Work out the finished part from the listing and answer in its coordinate system (mm). Round coordinates to 2 decimals unless told otherwise and drop trailing zeros. Loops run counter-clockwise (first coordinate to the right, second up) from the corner with the lowest first, then second, coordinate; pieces in that order, holes last. Notation, with made-up numbers: (75, -1.75) - (81, -1.75) arc R23 cw to (81, 37.25) - close; hole circle Ø8 at (-28, 52). An arc over 180 degrees is marked (long way). Return JSON: item names as keys, results as strings.
from build123d import *

# Parameters (mm, degrees)
F0_W     = 109
F0_H     = 70
F0_R     = 1.1
F0_R_2   = 6.3
F1_DEPTH = 1
F2_W     = 53
F2_H     = 10.5
F3_DEPTH = 1
F5_DEPTH = 1
F6_R     = 1
F7_R     = 1.1
F7_W     = 40
F7_H     = 16.5
F7_R_2   = 10
F8_DEPTH = 1
F9_R     = 3


# Not quite as in the source:
# - a feature names something its author has since deleted; it is built from what else it names


with BuildPart() as f1:
    # F0 (on Top) → F1 (new body)
    with BuildSketch(Plane.XY):
        Rectangle(F0_W, F0_H)
        with Locations((-51.5, -26)):
            Circle(F0_R, mode=Mode.SUBTRACT)
        with Locations((-35.5, -26)):
            Circle(F0_R, mode=Mode.SUBTRACT)
        with Locations((-23.5, -21.5)):
            Circle(F0_R, mode=Mode.SUBTRACT)
        with BuildLine():
            ThreePointArc((-37.5, -14.5), (-37.7928932188, -15.2071067812), (-38.5, -15.5))
            Line((-38.5, -15.5), (-48.5, -15.5))
            ThreePointArc((-48.5, -15.5), (-49.2071067812, -15.2071067812), (-49.5, -14.5))
            Line((-49.5, -14.5), (-49.5, -8.5))
            ThreePointArc((-49.5, -8.5), (-49.2071067812, -7.7928932188), (-48.5, -7.5))
            Line((-48.5, -7.5), (-38.5, -7.5))
            ThreePointArc((-38.5, -7.5), (-37.7928932188, -7.7928932188), (-37.5, -8.5))
            Line((-37.5, -8.5), (-37.5, -14.5))
        make_face(mode=Mode.SUBTRACT)
        with Locations((23.5, -21.5)):
            Circle(F0_R, mode=Mode.SUBTRACT)
        with Locations((35.5, -26)):
            Circle(F0_R, mode=Mode.SUBTRACT)
        with Locations((51.5, -26)):
            Circle(F0_R, mode=Mode.SUBTRACT)
        with BuildLine():
            Line((38.5, -7.5), (48.5, -7.5))
            ThreePointArc((48.5, -7.5), (49.2071067812, -7.7928932188), (49.5, -8.5))
            Line((49.5, -8.5), (49.5, -14.5))
            ThreePointArc((49.5, -14.5), (49.2071067812, -15.2071067812), (48.5, -15.5))
            Line((48.5, -15.5), (38.5, -15.5))
            ThreePointArc((38.5, -15.5), (37.7928932188, -15.2071067812), (37.5, -14.5))
            Line((37.5, -14.5), (37.5, -8.5))
            ThreePointArc((37.5, -8.5), (37.7928932188, -7.7928932188), (38.5, -7.5))
        make_face(mode=Mode.SUBTRACT)
        with Locations((-43.5, 3.5)):
            Circle(F0_R_2, mode=Mode.SUBTRACT)
        with Locations((-51.5, 10)):
            Circle(F0_R, mode=Mode.SUBTRACT)
        with Locations((-35.5, 10)):
            Circle(F0_R, mode=Mode.SUBTRACT)
        with Locations((-23.5, 21.5)):
            Circle(F0_R, mode=Mode.SUBTRACT)
        with Locations((43.5, 3.5)):
            Circle(F0_R_2, mode=Mode.SUBTRACT)
        with Locations((35.5, 10)):
            Circle(F0_R, mode=Mode.SUBTRACT)
        with Locations((51.5, 10)):
            Circle(F0_R, mode=Mode.SUBTRACT)
        with Locations((23.5, 21.5)):
            Circle(F0_R, mode=Mode.SUBTRACT)
    extrude(amount=F1_DEPTH)

    # F2 (on face) → F3 (cut, through all)
    with BuildSketch(Plane.XY.offset(1)):
        with BuildLine():
            Line((-26.5, 35), (-54.5, 35))
            Line((-54.5, 35), (-54.5, 13))
            Line((-54.5, 13), (-28.5, 13))
            ThreePointArc((-28.5, 13), (-27.0857864376, 13.5857864376), (-26.5, 15))
            Line((-26.5, 15), (-26.5, 24.5))
            Line((-26.5, 24.5), (-26.5, 35))
        make_face()
        with Locations((0, 29.75)):
            Rectangle(F2_W, F2_H)
        with BuildLine():
            Line((54.5, 35), (26.5, 35))
            Line((26.5, 35), (26.5, 24.5))
            Line((26.5, 24.5), (26.5, 15))
            ThreePointArc((26.5, 15), (27.0857864376, 13.5857864376), (28.5, 13))
            Line((28.5, 13), (54.5, 13))
            Line((54.5, 13), (54.5, 35))
        make_face()
    extrude(amount=-F3_DEPTH, mode=Mode.SUBTRACT)

    # F4 (on face) → F5 (cut, through all)
    with BuildSketch(Plane.XY.offset(1)):
        Polygon((-54.5, -29), (-54.5, -35), (0, -35), (54.5, -35), (54.5, -29), (0, -29), align=None)
    extrude(amount=-F5_DEPTH, mode=Mode.SUBTRACT)

    # F6
    f6_edges = [f1.edges().sort_by_distance(p)[0] for p in [
        (-54.5, -29, 0.5),
        (54.5, -29, 0.5),
        (54.5, 13, 0.5),
        (26.5, 24.5, 0.5),
        (-26.5, 24.5, 0.5),
        (-54.5, 13, 0.5),
    ]]
    fillet(f6_edges, radius=F6_R)

    # F7 (on face) → F8 (cut, through all)
    with BuildSketch(Plane.XY.offset(1)):
        with Locations((-22.5, -10)):
            Circle(F7_R)
        with Locations((22.5, -10)):
            Circle(F7_R)
        with Locations((-22.5, 12.5)):
            Circle(F7_R)
        with Locations((22.5, 12.5)):
            Circle(F7_R)
        with Locations((0, -20.75)):
            Rectangle(F7_W, F7_H)
        with Locations((0, 6)):
            Circle(F7_R_2)
    extrude(amount=-F8_DEPTH, mode=Mode.SUBTRACT)

    # F9
    f9_edges = [f1.edges().sort_by_distance(p)[0] for p in [
        (-20, -29, 0.5),
        (-20, -12.5, 0.5),
        (20, -12.5, 0.5),
        (20, -29, 0.5),
    ]]
    fillet(f9_edges, radius=F9_R)


solid = f1.part
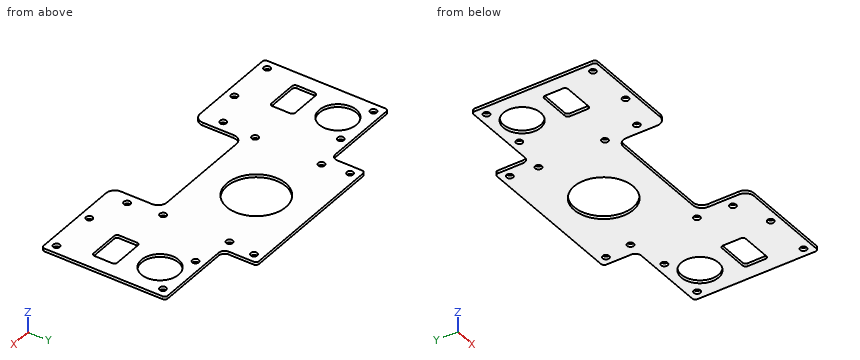
1) Section B-B (x = -51.5) is taken. Give the vertices of the cut face in (y, z).
Verdict:
{"outline": "(-29, 0) - (-27.1, 0) - (-27.1, 1) - (-29, 1) - close; (-24.9, 0) - (8.9, 0) - (8.9, 1) - (-24.9, 1) - close; (11.1, 0) - (13, 0) - (13, 1) - (11.1, 1) - close"}
2) Find the intervals of material crossed by L1, parallel to Y at x = 35.5, z = 0.75; L2, parallel to X at y = 22.5, z = 0.75; L3, parallel to X at y = -19, z = 0.9, in increasing order.
Verdict:
{"L1": "y = -29 to -27.1, -24.9 to 8.9, 11.1 to 13", "L2": "x = -26.5 to -23.96, -23.04 to 23.04, 23.96 to 26.5", "L3": "x = -54.5 to -20, 20 to 54.5"}
3) Section C-C (y = -17) is taken. Give the vertices of the cut face in (x, z), and give its area (3 significant figures).
Verdict:
{"outline": "(-54.5, 0) - (-20, 0) - (-20, 1) - (-54.5, 1) - close; (20, 0) - (54.5, 0) - (54.5, 1) - (20, 1) - close", "area": "69.0 mm2"}
4) Section D-D (y = 6) is taken. Give the vertices of the cut face in (x, z).
Verdict:
{"outline": "(-54.5, 0) - (-49.28, 0) - (-49.28, 1) - (-54.5, 1) - close; (-37.72, 0) - (-10, 0) - (-10, 1) - (-37.72, 1) - close; (10, 0) - (37.72, 0) - (37.72, 1) - (10, 1) - close; (49.28, 0) - (54.5, 0) - (54.5, 1) - (49.28, 1) - close"}
5) Flat-ended cylindrical pins translate along their axes: pin 1 (23 mm diameter, centred on x = 0, y = 6, fed in from +Z); pin 2 (0.5 mm diameter, centred on x = -45.5, z = 0.5, fed in from +Y). Find the tip coordinate at first contact, or state that the pin passes through.
Verdict:
{"pin 1": "stops at z = 1", "pin 2": "stops at y = 13"}
6) Section A-A (y = -10) is taken. Give the vertices of the cut face in (x, z), and give its area (3 significant figures).
Verdict:
{"outline": "(-54.5, 0) - (-49.5, 0) - (-49.5, 1) - (-54.5, 1) - close; (-37.5, 0) - (-23.6, 0) - (-23.6, 1) - (-37.5, 1) - close; (-21.4, 0) - (21.4, 0) - (21.4, 1) - (-21.4, 1) - close; (23.6, 0) - (37.5, 0) - (37.5, 1) - (23.6, 1) - close; (49.5, 0) - (54.5, 0) - (54.5, 1) - (49.5, 1) - close", "area": "80.6 mm2"}
